from build123d import *

# Parameters (mm, degrees)
BOSS_EXTRUDE1_START = 70
SKETCH2_R           = 32.5
BOSS_EXTRUDE1_DEPTH = 20
LPATTERN1_COUNT     = 2
LPATTERN1_PITCH     = 150
SKETCH4_R           = 10
BOSS_EXTRUDE2_DEPTH = 50


with BuildPart() as part:
    # Sketch1 → Revolve1 (revolve)
    with BuildSketch(Plane.XY, mode=Mode.PRIVATE) as revolve1_sk:
        Polygon((0, 248.5), (-32.5, 248.5), (-32.5, 45.5), (-24.5, 45.5), (-24.5, 27.5), (-6, 27.5), (-6, 0), (0, 0), align=None)
    revolve(revolve1_sk.sketch.rotate(Axis((0, 0, 0), (0, 1, 0)), 270), axis=Axis((0, 0, 0), (0, 1, 0)))

    # Sketch2 → Boss-Extrude1 (add)
    with BuildSketch(Plane(origin=(0, 0, 0), x_dir=(1, 0, 0), z_dir=(0, 1, 0)).offset(BOSS_EXTRUDE1_START)):
        with BuildLine():
            Line((-40, 0), (-40, 50))
            Line((-40, 50), (40, 50))
            Line((40, 50), (40, 0))
            ThreePointArc((40, 0), (0, -40), (-40, 0))
        make_face()
        with Locations(Location((0, 0, 0), (0, 0, 90))):
            Circle(SKETCH2_R, mode=Mode.SUBTRACT)
    boss_extrude1 = extrude(amount=BOSS_EXTRUDE1_DEPTH)

    # LPattern1: Boss-Extrude1 ×2
    with Locations(*[(0, i * LPATTERN1_PITCH, 0) for i in range(1, LPATTERN1_COUNT)]):
        add(boss_extrude1)

    # Sketch4 → Boss-Extrude2 (add)
    with BuildSketch(Plane.XZ):
        Circle(SKETCH4_R)
    extrude(amount=BOSS_EXTRUDE2_DEPTH)


solid = part.part
Read the model definition and answer for the solid it produces. Units are mm, in the model's axes. A direction names the side the tool comes from. Round coordinates to 2 decimals unless told otherwise and drop trailing zeros. Loops run counter-clockwise (first coordinate to the right, second up) from the corner with the lowest first, then second, coordinate; pieces in that order, holes last. Notation, with made-up numbers: (-16.75, -0.5) - (33.25, -0.5) arc R11 cw to (33.25, 15.5) - close; hole circle Ø3 at (15.5, 5). An arc over 180 degrees is marked (long way). One line per question, with ' | ' between items. Start each with the question number.
Q1. Find the intervals of material crossed by L1, parallel to Y at x = 19.5, z = -32.5; L2, parallel to Y at x = 29.5, z = 13.5; L3, parallel to Y at x = -20, z = -2, in increasing order.
Q2. Section B-B on y = 164 is taken. Give the vertices of the cut face in (x, z).
Q3. Flat-ended cylindrical pins translate along their axes: pin 1 (2 mm diameter, centred on y = 41, z = 15, fed in from +X); pin 2 (12 mm diameter, centred on x = 17.5, z = 24.5, fed in from -Y); pin 3 (5 mm diameter, centred on x = 1, y = 24.5, fed in from -Z); pin 4 (24 mm diameter, centred on x = -13, z = -11, fed in from -Y). Find the tip coordinate at first contact, or state that the pin passes through.
Q4. Section C-C on x = 17.5 is taken. Give the vertices of the cut face in (y, z), plus the area to 3 significant figures.
Q5. Section D-D on x = -29.5 is taken. Give the vertices of the cut face in (y, z), plus the area to 3 significant figures.
Q6. For faces 4 (the cylindrical face through (-9.76, 244.19, -31)), 5 (the flat face through (1, 70, -36)), 6 (the flat face through (0, 0, -7)), determine the directions among +Z, -Z, +X, -X, +Y, -Y from which every point of the face is accessible in a straight line to the end or side of a thin tool.
Q7. For a pull along Y with two mould halves and no side action, classify faces 1 (the flat face through (0, 248.5, 0)), 2 (the cylindrical face through (-1.802, 13.558, -5.723)), 3 (the flat face through (-40, 230, -25)) as +Y half, -Y half, draft (parallel to the pull), parting line (faces both ways), or undercut.
Established:
1) L1: 70 to 90, 220 to 240 | L2: 45.5 to 248.5 | L3: 27.5 to 248.5
2) outline: circle Ø65 at (0, 0)
3) pin 1: x = 20.11 | pin 2: y = 27.5 | pin 3: z = -6 | pin 4: y = -50
4) outline: (27.5, -17.15) - (45.5, -17.15) - (45.5, -27.39) - (70, -27.39) - (70, -50) - (90, -50) - (90, -27.39) - (220, -27.39) - (220, -50) - (240, -50) - (240, -27.39) - (248.5, -27.39) - (248.5, 27.39) - (240, 27.39) - (240, 35.97) - (220, 35.97) - (220, 27.39) - (90, 27.39) - (90, 35.97) - (70, 35.97) - (70, 27.39) - (45.5, 27.39) - (45.5, 17.15) - (27.5, 17.15) - close | area: 13,000 mm²
5) outline: (45.5, -13.64) - (70, -13.64) - (70, -50) - (90, -50) - (90, -13.64) - (220, -13.64) - (220, -50) - (240, -50) - (240, -13.64) - (248.5, -13.64) - (248.5, 13.64) - (240, 13.64) - (240, 27.01) - (220, 27.01) - (220, 13.64) - (90, 13.64) - (90, 27.01) - (70, 27.01) - (70, 13.64) - (45.5, 13.64) - close | area: 7,530 mm²
6) face 4: +Y | face 5: -Y | face 6: none
7) face 1: +Y half | face 2: undercut | face 3: draft
